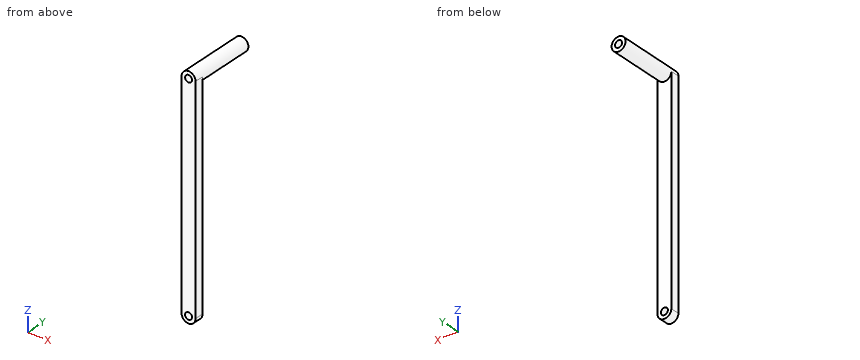
from build123d import *

# Parameters (mm, degrees)
SKETCH1_R           = 0.75
BOSS_EXTRUDE2_DEPTH = 2
SKETCH2_R           = 1.5
SKETCH2_R_2         = 0.75
BOSS_EXTRUDE3_DEPTH = 12.94


with BuildPart() as part:
    # Sketch1 → Boss-Extrude2 (new body)
    with BuildSketch(Plane(origin=(0, 0, 0), x_dir=(1, 0, 0), z_dir=(0, 1, 0))):
        with BuildLine():
            Line((0, 0), (0, 47))
            ThreePointArc((0, 47), (1.5, 48.5), (3, 47))
            Line((3, 47), (3, 0))
            ThreePointArc((3, 0), (1.5, -1.5), (0, 0))
        make_face()
        with Locations(Location((1.5, 0, 0), (0, 0, 270))):
            Circle(SKETCH1_R, mode=Mode.SUBTRACT)
        with Locations(Location((1.5, 47, 0), (0, 0, 270))):
            Circle(SKETCH1_R, mode=Mode.SUBTRACT)
    extrude(amount=BOSS_EXTRUDE2_DEPTH)

    # Sketch2 → Boss-Extrude3 (add)
    with BuildSketch(Plane(origin=(0, 2, 0), x_dir=(1, 0, 0), z_dir=(0, 1, 0))):
        with Locations((1.5, 0)):
            Circle(SKETCH2_R)
        with Locations(Location((1.5, 0, 0), (0, 0, 270))):
            Circle(SKETCH2_R_2, mode=Mode.SUBTRACT)
    extrude(amount=BOSS_EXTRUDE3_DEPTH)


solid = part.part
Build history of the part. All positions in model axes, mm. Round coordinates to 2 decimals unless told otherwise and drop trailing zeros. Loops run counter-clockwise (first coordinate to the right, second up) from the corner with the lowest first, then second, coordinate; pieces in that order, holes last. Notation, with made-up numbers: (89, -30) -> (96, -30) arc R16 ccw to (96, -6) -> close; hole circle Ø2 at (68.25, -4). An arc over 180 degrees is marked (long way). Answer in a Markdown table with one row per item.
Item 1: Saw through at A-A (x = 1.5). Write the cut outline in (y, z), and give its area (3 significant figures).
Answers below:
| item | result |
|---|---|
| outline | (0, -48.5) -> (2, -48.5) -> (2, -47.75) -> (0, -47.75) -> close; (0, -46.25) -> (2, -46.25) -> (2, -1.5) -> (14.94, -1.5) -> (14.94, -0.75) -> (0, -0.75) -> close; (0, 0.75) -> (14.94, 0.75) -> (14.94, 1.5) -> (0, 1.5) -> close |
| area | 113 mm² |
Item 2: Drill centre lines: L1, parallel to X at y = 8.75, z = 0; L2, parallel to Z at x = 0.2, y = 2.5; L3, parallel to Y at x = 1.25, z = -27. Where is each one in solid material? Low to high. Write a range as [from, to].
Answers below:
| item | result |
|---|---|
| L1 | x = [0, 0.75], [2.25, 3] |
| L2 | z = [-0.75, 0.75] |
| L3 | y = [0, 2] |
Item 3: Pin check, flat tips, straight feed: pin 1 (1.2 mm diameter, centred on x = 1.5, z = -47, fed in from +Y); pin 2 (1 mm diameter, centred on x = 2, z = -33.5, fed in from +Y). Stop position of each tip, or through.
Answers below:
| item | result |
|---|---|
| pin 1 | passes through |
| pin 2 | stops at y = 2 |
Item 4: Saw through at B-B (y = 7.75). Write the cut outline in (x, z).
Answers below:
| item | result |
|---|---|
| outline | circle Ø3 at (1.5, 0); hole circle Ø1.5 at (1.5, 0) |
Item 5: Saw through at C-C (z = -33.5). Write the cut outline in (x, y).
Answers below:
| item | result |
|---|---|
| outline | (0, 0) -> (3, 0) -> (3, 2) -> (0, 2) -> close |
